For this review, take the finished solid that the model builds, in its own axes (mm). A direction names the side the tool comes from. Give positions to 0.01 mm unless a question says otherwise; leave off trailing zeros. Write each loop counter-clockwise with the first axis right and the second up, starting at its lowest first coordinate (ties: lowest second). Pieces come first, ordered by that corner, then holes.
1) Machinability: for faces 1 (the face through (42, 10, 51)), 2 (the face through (62, 3, 25)), 3 (the face through (21, 6, 47)), which of the approach directions +Z, -Z, +X, -X, +Y, -Y give a long, thin tool a straight path to every point of the face, cutting with its end or side? Answer none if there is none.
2) We need section D-D on y = 4.5. Give the boundary of the cut face in (x, z), and give its area (3 significant figures).
3) For P1, Ø6.5, axis at x = 36.5, y = 5.5, coming from the -Z side; P2, Ø4.5, axis at y = 10, z = 52, coming from the +X side; P3, Ø2.5, axis at x = 5.5, y = 5.5, coming from the +Z side; P4, Ø14.5, axis at x = 54, z = 18.5, coming from the +Y side, all flat-tipped, find the tip position at first contact; note any pin that passes through.
4) Wall thickness on line 1 along Z through (x, y) = (17, 7.25); line 2 along Y through (x, z) = (36.5, 51.25); line 3 along Y through (x, z) = (36, 49): over which ranges is each line inside the solid? List them lowest first.
5) We need section A-A on x = 36.5. Give the boundary of the cut face in (y, z), and give its area (3 significant figures).
6) We need section B-B on y = 11. Give the boundary of the cut face in (x, z), and give its area (3 significant figures).
7) We need section C-C on z = 38. Give the boundary of the cut face in (x, y).
Autodesk Inventor part; units mm, degrees
ref_plane "Work Plane1" through (21, 21, 47) normal (0, 0, 1) x (1, 0, 0)
ref_plane "Work Plane2" through (0, 3.5, 0) normal (-1, 0, 0) x (0, 0, 1)
ref_plane "YZ Plane" through (0, 0, 0) normal (1, 0, 0) x (0, 1, 0)
ref_plane "Work Plane1" through (21, 21, 47) normal (0, 0, 1) x (1, 0, 0)
sketch "Sketch1" plane through (21, 21, 47) normal (0, 0, 1) x (1, 0, 0)
  line L0 (21, -17.5) -> (21, 17.5) construction
  line L1 (-17.5, -21) -> (17.5, -21) construction
  line L2 (21, -21) -> (9, -21)
  line L3 (9, -21) -> (9, -9)
  line L4 (9, -9) -> (21, -9)
  line L5 (21, -9) -> (21, -21)
  point P0 (-21, -21)
  dimension "d0" = 12
  dimension "d1" = 12
extrude "Extrusion1" add sketch "Sketch1" along normal blind 8
sketch "Sketch2" plane through (42, 0, 47) normal (1, 0, 0) x (0, 0, -1)
  line L0 (-8, 0) -> (0, 0)
  line L1 (0, 0) -> (0, 5)
  line L2 (0, 5) -> (-8, 5)
  line L3 (-8, 5) -> (-8, 0)
  point P0 (47, 0)
  dimension "d4" = 8
  dimension "d5" = 5
extrude "Extrusion2" add sketch "Sketch2" along normal blind 20
sketch "Sketch3" plane through (21, 21, 47) normal (0, 0, -1) x (-1, 0, 0)
  line L0 (-41, -16) -> (-22, -16)
  line L1 (-22, -16) -> (-22, -21)
  line L2 (-22, -21) -> (-41, -21)
  line L3 (-41, -21) -> (-41, -16)
  point P0 (21, -21)
  dimension "d8" = 19
  dimension "d9" = 5
extrude "Extrusion3" add sketch "Sketch3" along normal blind 20
sketch "Sketch4" plane through (21, 21, 55) normal (0, 0, 1) x (1, 0, 0)
  circle A0 centre (15.5, -15.5) radius 1.5
  circle A1 centre (15.5, -15.5) radius 2
  point P0 (-21, -21)
  dimension "d15" = 0.5
extrude "Extrusion4" cut sketch "Sketch4" against normal blind 8 contours A0 | A1
sketch "Sketch5" plane through (30, 0, 47) normal (-1, 0, 0) x (0, 0, 1)
  line L0 (0, 0) -> (0, 12)
  line L1 (0, 0) -> (8, 0)
  line L2 (8, 12) -> (8, 0)
  line L3 (0, 12) -> (8, 12)
  point P0 (-47, 0)
ref_plane "Work Plane2" through (0, 3.5, 0) normal (-1, 0, 0) x (0, 0, 1)
extrude "Extrusion5" add sketch "Sketch5" along normal up to surface (30 mm away)
sketch "Sketch6" plane through (21, 21, 55) normal (0, 0, 1) x (1, 0, 0)
  circle A0 centre (-15.5, -15.5) radius 1.5
  circle A1 centre (-15.5, -15.5) radius 2
  dimension "d20" = 0.5
extrude "Extrusion6" cut sketch "Sketch6" against normal blind 8 contours A0 | A1
sketch "Sketch7" plane through (21, 21, 55) normal (0, 0, 1) x (1, 0, 0)
  line L0 (21, -9) -> (-21, -9)
  circle A0 centre (0, 0) radius 11
  arc A1 (-10.1679, -9) -> (10.1679, -9) centre (0, 0) ccw
  line L1 (-10.1679, -9) -> (11.2714, -9)
  line L2 (-13.5789, -9) -> (17.965, -9)
extrude "Extrusion7" cut sketch "Sketch7" against normal blind 8 contours A1 L0 A0 | A0 L0 picked at (-1.3175, -9.4218)
sketch "Sketch8" plane through (21, 21, 55) normal (0, 0, 1) x (1, 0, 0)
  line L0 (-21, -9) -> (-21, -21)
  line L1 (41, -21) -> (-21, -21)
  line L2 (-17.5, -21) -> (-21, -17.5)
extrude "Extrusion8" cut sketch "Sketch8" against normal blind 8
fillet "Fillet4" radius 5 1 edges at (62, 2.5, 55)
sketch "Sketch10" plane through (21, 21, 27) normal (0, 0, -1) x (-1, 0, 0)
  line L0 (-41, -16) -> (-41, -21)
  line L1 (-41, -21) -> (-22, -21)
  line L2 (-22, -21) -> (-22, -16)
  line L3 (-22, -16) -> (-41, -16)
  point P0 (21, -21)
extrude "Extrusion10" add sketch "Sketch10" along normal blind 27
sketch "Sketch11" plane through (42, 5, 55) normal (0, 1, 0) x (1, 0, 0)
  arc A0 (15, 0) -> (20, 5) centre (15, 5) ccw
  line L0 (20, 5) -> (20, 55)
  line L1 (1, 55) -> (20, 55)
  line L2 (1, 8) -> (1, 55)
  line L3 (0, 8) -> (1, 8)
  line L4 (0, 0) -> (0, 8)
  line L5 (0, 0) -> (15, 0)
  point P0 (-42, 55)
extrude "Extrusion11" add sketch "Sketch11" along normal blind 1
fillet "Fillet5" radius 2 1 edges at (42, 6, 51)
properties part number "RightBracket"
Results list:
1. face 1: +Z, -Z, +X, +Y
1. face 2: +Z, -Z, +X, +Y, -Y
1. face 3: -Z, -X, +Y, -Y
2. outline: (0, 47) - (3.77, 47) - (3.77, 55) - (0, 55) - close; (7.23, 47) - (34.77, 47) - (34.77, 55) - (7.23, 55) - close; (38.23, 47) - (43, 47) - (43, 0) - (62, 0) - (62, 50) arc R5 ccw to (57, 55) - (38.23, 55) - close
2. area: 1,330 mm2
3. P1: stops at z = 47
3. P2: stops at x = 42.02
3. P3: passes through
3. P4: stops at y = 6
4. line 1: z = 47 to 55
4. line 2: y = 0 to 3.5, 7.5 to 12
4. line 3: y = 0 to 3.56, 7.44 to 12
5. outline: (0, 47) - (3.5, 47) - (3.5, 55) - (0, 55) - close; (7.5, 47) - (12, 47) - (12, 55) - (7.5, 55) - close
5. area: 64.0 mm2
6. outline: (0, 47) - (11.81, 47) - (11.81, 55) - (0, 55) - close; (30.19, 47) - (42, 47) - (42, 55) - (30.19, 55) - close
6. area: 189 mm2
7. outline: (43, 0) - (62, 0) - (62, 6) - (44, 6) arc R2 cw to (43, 6.27) - close
